from build123d import *

# Parameters (mm, degrees)
SKETCH1_W           = 174
SKETCH1_H           = 78
SKETCH1_R           = 34
SKETCH1_R_2         = 2.5
BOSS_EXTRUDE1_DEPTH = 10


with BuildPart() as part:
    # Sketch1 → Boss-Extrude1 (new body)
    with BuildSketch(Plane(origin=(0, 0, 0), x_dir=(1, 0, 0), z_dir=(0, 1, 0))):
        Rectangle(SKETCH1_W, SKETCH1_H)
        with Locations(Location((48, 0, 0), (0, 0, 270))):
            Circle(SKETCH1_R, mode=Mode.SUBTRACT)
        with Locations(Location((-48, 0, 0), (0, 0, 270))):
            Circle(SKETCH1_R, mode=Mode.SUBTRACT)
        with Locations(Location((-79.5, 31.5, 0), (0, 0, 270))):
            Circle(SKETCH1_R_2, mode=Mode.SUBTRACT)
        with Locations(Location((-79.5, -31.5, 0), (0, 0, 270))):
            Circle(SKETCH1_R_2, mode=Mode.SUBTRACT)
        with Locations(Location((79.5, -31.5, 0), (0, 0, 270))):
            Circle(SKETCH1_R_2, mode=Mode.SUBTRACT)
        with Locations(Location((79.5, 31.5, 0), (0, 0, 270))):
            Circle(SKETCH1_R_2, mode=Mode.SUBTRACT)
        with BuildLine():
            ThreePointArc((-5.678908346, 10), (0, -11.5), (5.678908346, 10))
            ThreePointArc((5.678908346, 10), (0, 31.5), (-5.678908346, 10))
        make_face(mode=Mode.SUBTRACT)
    extrude(amount=BOSS_EXTRUDE1_DEPTH)


solid = part.part
Source: CAD feature listing. Evaluate the final solid. Frame: model axes, mm. Round coordinates to 2 decimals unless told otherwise and drop trailing zeros. Write each loop counter-clockwise with the first axis right and the second up, starting at its lowest first coordinate (ties: lowest second). Pieces come first, ordered by that corner, then holes. Notation, with made-up numbers: (2, 67.5) - (43, 67.5) arc R14 cw to (43, 86.5) - close; hole circle Ø3 at (-19, 65). An arc over 180 degrees is marked (long way). Use CSV: the item, a comma, the result in double quotes. Start each with the question number.
(1) Mould query, pull axis Z, two halves, no side actions, for faces 1 (the face through (79.6, 4.9, -34)), 2 (the face through (-79.4, 4.9, -34)), 3 (the face through (87, 5, 1)), 4 (the face through (-1, 5, 39)). Classes: pulls with the +Z half, pulls with the -Z half, needs draft (parallel to the pull), parting line crosses it, or undercut.
(2) Cut plane C-C, the plane x = 79.5. Return loops of the section in (y, z), and give its area (3 significant figures).
(3) Cut plane B-B, the plane z = 0. Return loops of the section in (x, y), and give its area (3 significant figures).
(4) Material intervals for probe 1 along X at (y, z) = (6, 0); probe 2 along X at (y, z) = (3, 6.5); probe 3 along X at (y, z) = (7.75, 20.5), sorted ascending. Write a range as [from, to].
(5) Cut plane A-A, the plane x = 48. Return loops of the section in (y, z).
(6) Cut plane D-D, the plane z = 26.5. Return loops of the section in (x, y).
Geometry says:
1,face 1,"undercut"
1,face 2,"undercut"
1,face 3,"needs draft"
1,face 4,"pulls with the +Z half"
2,outline,"(0, -39) - (10, -39) - (10, -34) - (0, -34) - close; (0, -29) - (10, -29) - (10, -12.8) - (0, -12.8) - close; (0, 12.8) - (10, 12.8) - (10, 29) - (0, 29) - close; (0, 34) - (10, 34) - (10, 39) - (0, 39) - close"
2,area,"424 mm²"
3,outline,"(-87, 0) - (-82, 0) - (-82, 10) - (-87, 10) - close; (-14, 0) - (-11.5, 0) - (-11.5, 10) - (-14, 10) - close; (11.5, 0) - (14, 0) - (14, 10) - (11.5, 10) - close; (82, 0) - (87, 0) - (87, 10) - (82, 10) - close"
3,area,"150 mm²"
4,probe 1,"[-87, -82], [-14, -11.5], [11.5, 14], [82, 87]"
4,probe 2,"[-87, -81.37], [-14.63, -9.49], [9.49, 14.63], [81.37, 87]"
4,probe 3,"[-87, -75.12], [-20.88, 20.88], [75.12, 87]"
5,outline,"(0, -39) - (10, -39) - (10, -34) - (0, -34) - close; (0, 34) - (10, 34) - (10, 39) - (0, 39) - close"
6,outline,"(-87, 0) - (-69.3, 0) - (-69.3, 10) - (-87, 10) - close; (-26.7, 0) - (26.7, 0) - (26.7, 10) - (-26.7, 10) - close; (69.3, 0) - (87, 0) - (87, 10) - (69.3, 10) - close"
